```python
from build123d import *

# Parameters (mm, degrees)
F0_W        = 127
F0_H        = 76.2
F1_DEPTH    = 12.7
F2_R        = 6.35
F3_DEPTH    = 12.701
F4_W        = 12.7
F4_H        = 50.8
F6_W        = 13.0245922636
F6_H        = 6.35
F8_R        = 5.08
F9_T1_DEPTH = 140.0641495789
F9_T3_DEPTH = 89.2641495789


# Not quite as in the source:
# - a fillet or chamfer that OpenCascade refuses, or shapes differently, is made with other operations: its cross-section is extruded or revolved along the edge and cut away or added


with BuildPart() as f1:
    # F0 (on Top) → F1 (new body)
    with BuildSketch(Plane.XY):
        Rectangle(F0_W, F0_H)
    extrude(amount=F1_DEPTH)

    # F2 (on face) → F3 (cut, through all)
    with BuildSketch(Plane.XY.offset(12.7)):
        with Locations((-52.3479245603, 27.9940944165)):
            Circle(F2_R)
        with Locations((53.7015721202, 29.8446007073)):
            Circle(F2_R)
        with Locations((-50.5206361413, -27.9734656215)):
            Circle(F2_R)
        with Locations((53.327344358, -29.6574886888)):
            Circle(F2_R)
    extrude(amount=-F3_DEPTH, mode=Mode.SUBTRACT)

    # F4 (on Front) → F5 (revolve)
    with BuildSketch(Plane.XZ):
        with Locations((6.35, 38.1)):
            Rectangle(F4_W, F4_H)
    revolve(axis=Axis((0, 0, 38.1), (0, 0, 1)))

    # F6 (on Front) → F7 (revolve, cut)
    with BuildSketch(Plane.XZ):
        with Locations((16.6722961318, 41.275)):
            Rectangle(F6_W, F6_H)
    revolve(axis=Axis((0, 0, 38.1), (0, 0, 1)), mode=Mode.SUBTRACT)

    # F8
    f8_edges = [f1.edges().sort_by_distance(p)[0] for p in [
        (-12.7, 0, 63.5),
        (-12.7, 0, 12.7),
    ]]
    fillet(f8_edges, radius=F8_R)

    # F9: chamfer of 2.54 on 4 edges, made by hand

    # F9_s2 → F9_t1 (cut)
    with BuildSketch(Plane.YZ.offset(-70.0320747894)):
        Polygon((-35.56, 12.7), (-38.1, 10.16), (-38.1, 12.7), align=None)
        Polygon((35.56, 12.7), (38.1, 10.16), (38.1, 12.7), align=None)
    extrude(amount=F9_T1_DEPTH, mode=Mode.SUBTRACT)

    # F9_s4 → F9_t3 (cut)
    with BuildSketch(Plane.XZ.offset(-44.6320747894)):
        Polygon((60.96, 12.7), (63.5, 10.16), (63.5, 12.7), align=None)
        Polygon((-60.96, 12.7), (-63.5, 10.16), (-63.5, 12.7), align=None)
    extrude(amount=F9_T3_DEPTH, mode=Mode.SUBTRACT)


solid = f1.part
```
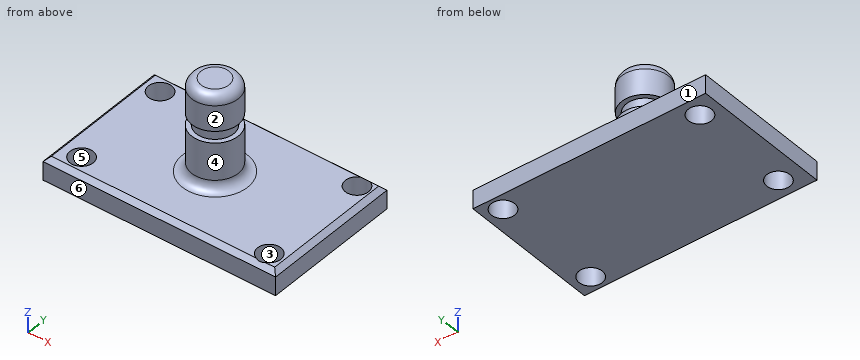
For this review, take the finished solid that the model builds, in its own axes (mm). Face numbers are marked on the shaded views. A direction names the side the tool comes from. Give positions to 0.01 mm unless a question says otherwise; leave off trailing zeros. Loops run counter-clockwise (first coordinate to the right, second up) from the corner with the lowest first, then second, coordinate; pieces in that order, holes last. Notation, with made-up numbers: M 55.5,33.25 L 114.5,33.25 A33 cw 114.5,67.25 Z; hole C -21,32 d7. An arc over 180 degrees is marked long. One line per item, written item: value. Start each with the question number.
Q1. Add section C-C (z = 5.5). Give the boundary of the cut face in (x, y).
Q2. Add section B-B (x = 0). Give the boundary of the cut face in (y, z).
Q3. Add section D-D (y = -26). Give the boundary of the cut face in (x, z).
Q4. For L1, parallel to Z at x = 37.5, y = -34; L2, parallel to X at y = -8.5, z = 10.5; L3, parallel to X at y = 3, z = 29.5, list the stretches that pass through material, from the lowest coordinate up.
Q5. Clearance check with flat-ended pins moving along their axes: pin 1 Ø11.5 at (x, y) = (53.7, 29.84) entering from -Z; pin 2 Ø1.5 at (x, y) = (23.5, -6) entering from +Z; pin 3 Ø1.5 at (x, y) = (15.5, 21.5) entering from -Z; pin 4 Ø1.5 at (x, z) = (38.5, 12) entering from +Y. State where each tip first meets the part, or that it passes through.
Q6. Machinability: for the marked faces 1 and 2, which of the approach directions +Z, -Z, +X, -X, +Y, -Y give a long, thin tool a straight path to every point of the face, cutting with its end or side? Answer none if there is none.
Q7. Add section A-A (y = 0). Give the boundary of the cut face in (x, z), and give its area (3 significant figures).
Q8. Draft analysis for pull direction X (two halves, no side actions). For the marked faces 3, 4, 5 and 6, state which applies: released by +X, released by -X, zero draft, split by the parting line, or undercut.
Reply:
1. outline: M -63.5,-38.1 L 63.5,-38.1 L 63.5,38.1 L -63.5,38.1 Z; hole C -52.35,27.99 d12.7; hole C -50.52,-27.97 d12.7; hole C 53.33,-29.66 d12.7; hole C 53.7,29.84 d12.7
2. outline: M -38.1,0 L 38.1,0 L 38.1,10.16 L 35.56,12.7 L 17.78,12.7 A5.08 cw 12.7,17.78 L 12.7,38.1 L 10.16,38.1 L 10.16,44.45 L 12.7,44.45 L 12.7,58.42 A5.08 ccw 7.62,63.5 L -7.62,63.5 A5.08 ccw -12.7,58.42 L -12.7,44.45 L -10.16,44.45 L -10.16,38.1 L -12.7,38.1 L -12.7,17.78 A5.08 cw -17.78,12.7 L -35.56,12.7 L -38.1,10.16 Z
3. outline: M -63.5,0 L -56.56,0 L -56.56,12.7 L -60.96,12.7 L -63.5,10.16 Z; M -44.49,0 L 48.14,0 L 48.14,12.7 L -44.49,12.7 Z; M 58.52,0 L 63.5,0 L 63.5,10.16 L 60.96,12.7 L 58.52,12.7 Z
4. L1: 0 to 12.7
4. L2: -63.16 to 63.16
4. L3: -12.34 to 12.34
5. pin 1: through
5. pin 2: z = 12.7
5. pin 3: z = 0
5. pin 4: y = 37.01
6. face 1: +Z, -Z, +X, -X, +Y
6. face 2: +Z
7. outline: M -63.5,0 L 63.5,0 L 63.5,10.16 L 60.96,12.7 L 17.78,12.7 A5.08 cw 12.7,17.78 L 12.7,38.1 L 10.16,38.1 L 10.16,44.45 L 12.7,44.45 L 12.7,58.42 A5.08 ccw 7.62,63.5 L -7.62,63.5 A5.08 ccw -12.7,58.42 L -12.7,44.45 L -10.16,44.45 L -10.16,38.1 L -12.7,38.1 L -12.7,17.78 A5.08 cw -17.78,12.7 L -60.96,12.7 L -63.5,10.16 Z
7. area: 2,860 mm²
8. face 3: undercut
8. face 4: split by the parting line
8. face 5: undercut
8. face 6: zero draft
